Verification items for this drawing (mm, ordinates from the low corner). Coordinates: 2 decimals unless noted, no trailing zeros. Loops run counter-clockwise (first coordinate to the right, second up) from the corner with the lowest first, then second, coordinate; pieces in that order, holes last. Notation, with made-up numbers: M -12,-28.5 L 34,-28.5 A17 ccw 34,-2.5 Z; hole C -40,80.5 d3. An arc over 180 degrees is marked long. Return JSON: item names as keys, results as strings.
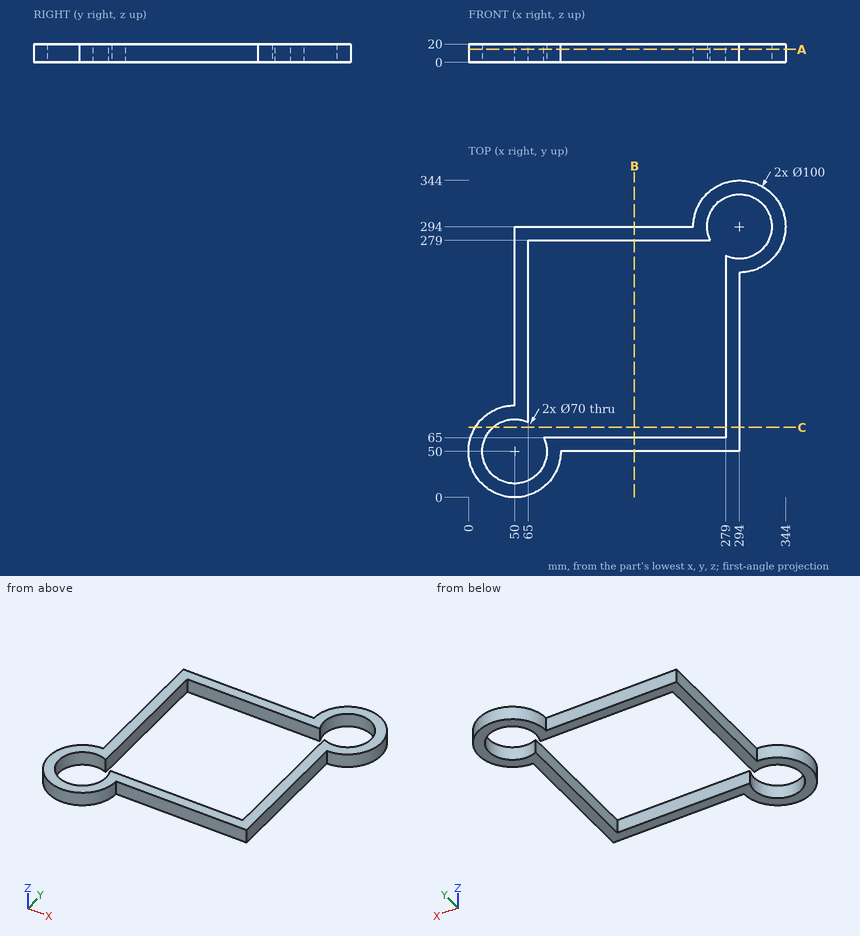
1) Go/stop test with flat-tipped pins: pin 1 Ø6 at (y, z) = (135, 6) entering from +X; pin 2 Ø1 at (x, z) = (240.5, 9) entering from -Y; pin 3 Ø6 at (x, z) = (143, 11.5) entering from +Y. Record where each tip stops, or that it passes through.
Answers:
{"pin 1": "x = 294", "pin 2": "y = 50", "pin 3": "y = 294"}
2) Section check A-A on z = 14.25. Record the cut outline in (x, y), then the cut area to 3 significant figures.
Answers:
{"outline": "M 50,100 A50 ccw long 100,50 L 294,50 L 294,244 A50 ccw long 244,294 L 50,294 Z; hole M 65,81.62 A35 ccw long 81.62,65 L 279,65 L 279,262.38 A35 ccw long 262.38,279 L 65,279 Z", "area": "18,200 mm²"}
3) Scan lines: line 1 along X through (y, z) = (224, 18); line 2 along X through (y, z) = (268.5, 13.75). Record each from-to range of solid material in increasing order. Write a range as [from, to].
Answers:
{"line 1": "[50, 65], [279, 294]", "line 2": "[50, 65], [317.97, 337.01]"}
4) Section check B-B on x = 180. Record the cut outline in (y, z), then the cut area to 3 significant figures.
Answers:
{"outline": "M 50,0 L 65,0 L 65,20 L 50,20 Z; M 279,0 L 294,0 L 294,20 L 279,20 Z", "area": "600 mm²"}
5) Section check C-C on y = 76. Record the cut outline in (x, z).
Answers:
{"outline": "M 7.29,0 L 26.57,0 L 26.57,20 L 7.29,20 Z; M 279,0 L 294,0 L 294,20 L 279,20 Z"}
